Autodesk Inventor part; units mm, degrees
ref_plane "Work Plane1" through (-15.3416, 0, -12.2936) normal (1, 0, 0) x (0, 0, -1)
ref_plane "Work Plane2" through (-24.8666, 0, -12.2936) normal (1, 0, 0) x (0, 0, -1)
ref_plane "YZ Plane" through (0, 0, 0) normal (1, 0, 0) x (0, 1, 0)
sketch "Sketch1" plane through (0, 0, 0) normal (0, 1, 0) x (-1, 0, 0)
  line L0 (0, 0) -> (30.0482, 0)
  line L1 (30.0482, 0) -> (30.0482, -24.13)
  line L2 (30.0482, -24.13) -> (0, -24.13)
  line L3 (0, -24.13) -> (0, 0)
  line L4 (15.3416, -12.2936) -> (15.3416, -20.8026) construction
  line L5 (13.9319, -12.2936) -> (13.9319, -20.8026)
  line L6 (16.7513, -20.8026) -> (16.7513, -12.2936)
  arc A0 (16.7513, -12.2936) -> (13.9319, -12.2936) centre (15.3416, -12.2936) ccw
  arc A1 (13.9319, -20.8026) -> (16.7513, -20.8026) centre (15.3416, -20.8026) ccw
  line L7 (24.8666, -12.2936) -> (24.8666, -20.8026) construction
  line L8 (23.4569, -12.2936) -> (23.4569, -20.8026)
  line L9 (26.2763, -20.8026) -> (26.2763, -12.2936)
  arc A2 (26.2763, -12.2936) -> (23.4569, -12.2936) centre (24.8666, -12.2936) ccw
  arc A3 (23.4569, -20.8026) -> (26.2763, -20.8026) centre (24.8666, -20.8026) ccw
  line L10 (26.4414, -4.4958) -> (3.6068, -4.4958) construction
  line L11 (26.4414, -2.7958) -> (3.6068, -2.7958)
  line L12 (3.6068, -6.1958) -> (26.4414, -6.1958)
  arc A4 (26.4414, -6.1958) -> (26.4414, -2.7958) centre (26.4414, -4.4958) ccw
  arc A5 (3.6068, -2.7958) -> (3.6068, -6.1958) centre (3.6068, -4.4958) ccw
  point P0 (15.3416, -16.5481)
  point P1 (24.8666, -16.5481)
  point P2 (15.0241, -4.4958)
  dimension "d0" = 30.0482
  dimension "d1" = 24.13
  dimension "d5" = 12.2936
  dimension "d6" = 2.8194
  dimension "d8" = 3.3274
  dimension "d11" = 9.525
  dimension "d16" = 3.4
  dimension "d17" = 4.4958
  dimension "d18" = 3.6068
  dimension "d19" = 3.6068
  dimension "d43" = 5.1816
extrude "Shape" add sketch "Sketch1" along normal blind 2.54
sketch "Sketch2" plane through (0, 2.54, 0) normal (0, 1, 0) x (1, 0, 0)
  line L0 (0, 24.13) -> (-30.0482, 24.13)
  line L1 (0, 0) -> (0, 24.13)
  line L2 (-30.0482, 24.13) -> (0, 24.13)
  line L3 (0, 24.13) -> (0, 9.5)
  line L4 (0, 9.5) -> (-30.0482, 9.5)
  line L5 (-30.0482, 9.5) -> (-30.0482, 24.13)
  line L6 (-30.0482, 0) -> (0, 0)
  line L7 (-11.9634, 9.5) -> (-11.9634, 24.13)
  line L8 (-11.9634, 24.13) -> (-18.6944, 24.13)
  line L9 (-18.6944, 24.13) -> (-18.6944, 9.5)
  arc A0 (-16.7513, 12.2936) -> (-13.9319, 12.2936) centre (-15.3416, 12.2936) ccw
  line L10 (-18.1778, 2.3562) -> (-11.9634, 24.13) construction
  line L11 (-12.9982, 4.0205) -> (-18.6944, 24.13) construction
  line L12 (-18.6944, 9.5) -> (-1.5875, 9.5)
  line L13 (-28.2194, 24.13) -> (-28.2194, 9.5)
  line L14 (-21.4884, 9.5) -> (-21.4884, 24.13)
  line L15 (-28.2194, 9.5) -> (-11.1125, 9.5)
  line L16 (-21.4884, 24.13) -> (-28.2194, 24.13)
  point P0 (-11.9634, 24.13)
  point P1 (-21.4884, 9.5)
  point P2 (-18.6944, 9.5)
  point P3 (-28.2194, 24.13)
  dimension "d22" = 9.5
  dimension "d23" = 6.731
  dimension "d27" = 9.525
  dimension "d44" = 1.8288
extrude "Extrusion2" add sketch "Sketch2" along normal blind 3.937 contours L1 L4 L7 L0 | L9 L4 L14 L0 | L13 L4 L5 L0
ref_plane "Work Plane1" through (-15.3416, 0, -12.2936) normal (1, 0, 0) x (0, 0, -1)
ref_plane "Work Plane2" through (-24.8666, 0, -12.2936) normal (1, 0, 0) x (0, 0, -1)
sketch "Sketch3" plane through (0, 0, 0) normal (1, 0, 0) x (0, 0, -1)
  line L0 (24.13, 6.477) -> (9.5, 6.477)
  line L1 (24.13, 6.477) -> (21.59, 6.477)
  line L2 (21.59, 6.477) -> (21.59, 5.207)
  line L3 (21.59, 5.207) -> (24.13, 5.207)
  line L4 (24.13, 5.207) -> (24.13, 6.477)
  point P0 (0, 0)
  dimension "d35" = 2.54
  dimension "d36" = 1.27
extrude "Extrusion3" cut sketch "Sketch3" against normal through all
fillet "Fillet2" radius 3.175 4 edges at (0, 1.27, 0) (0, 2.6035, -24.13) (-30.0482, 2.6035, -24.13) (-30.0482, 1.27, 0)
equation "\"d19\" = d18"
equation "\"d27\" = d11"
properties part number "Limit switch mount top nut well"
CAD build for the part. Positions are in the model's coordinates, mm. A direction names the side the tool comes from. Give positions to 0.01 mm unless a question says otherwise; leave off trailing zeros. Loops run counter-clockwise (first coordinate to the right, second up) from the corner with the lowest first, then second, coordinate; pieces in that order, holes last. Notation, with made-up numbers: M -40,19 L -31,19 A22 cw -31,25 Z; hole C 33,-15 d8. An arc over 180 degrees is marked long. Write each question's results on one line, items separated by ' | '.
Q1. Band-saw the part on D-D on y = 1.25. Write the cut outline in (x, z) (3 decimals), and give its area (3 significant figures).
Geometry check:
outline: M -30.048,-20.955 A3.175 ccw -26.873,-24.13 L -3.175,-24.13 A3.175 ccw 0,-20.955 L 0,-3.175 A3.175 ccw -3.175,0 L -26.873,0 A3.175 ccw -30.048,-3.175 Z; hole M -26.441,-6.196 L -3.607,-6.196 A1.7 ccw -3.607,-2.796 L -26.441,-2.796 A1.7 ccw Z; hole M -26.276,-20.803 A1.41 ccw -23.457,-20.803 L -23.457,-12.294 A1.41 ccw -26.276,-12.294 Z; hole M -16.751,-20.803 A1.41 ccw -13.932,-20.803 L -13.932,-12.294 A1.41 ccw -16.751,-12.294 Z | area: 569 mm²
Q2. Band-saw the part on B-B on z = -16.75. Write the cut outline in (x, y).
Geometry check:
outline: M -30.05,0 L -26.28,0 L -26.28,2.54 L -28.22,2.54 L -28.22,6.48 L -30.05,6.48 Z; M -23.46,0 L -16.75,0 L -16.75,2.54 L -18.69,2.54 L -18.69,6.48 L -21.49,6.48 L -21.49,2.54 L -23.46,2.54 Z; M -13.93,0 L 0,0 L 0,6.48 L -11.96,6.48 L -11.96,2.54 L -13.93,2.54 Z
Q3. Flat gauge pins, fed straight in: P1, Ø2, axis at x = -9, z = -23, coming from the +Y side; P2, Ø0.6, axis at x = -29, y = 6, coming from the -Z side; P3, Ø1.4, axis at x = -20, y = 5, coming from the +Z side. Where does each tip first touch, or does it go through?
Geometry check:
P1: stops at y = 5.21 | P2: stops at z = -21.59 | P3: stops at z = -9.5
Q4. Band-saw the part on A-A on x = -22. Write the cut outline in (y, z), and give its area (3 significant figures).
Geometry check:
outline: M 0,-24.13 L 2.54,-24.13 L 2.54,-6.2 L 0,-6.2 Z; M 0,-2.8 L 2.54,-2.8 L 2.54,0 L 0,0 Z | area: 52.7 mm²
Q5. Mould opens along X. For faces 6 (the face through (-18.694, 4, -17)), 7 (the face through (0, 3, -14)), 8 (the face through (-29, 6.477, -16)) say: pulls with the +X half, pulls with the -X half, needs draft (parallel to the pull), parting line crosses it, or undercut.
Geometry check:
face 6: undercut | face 7: pulls with the +X half | face 8: needs draft
Q6. Band-saw the part on C-C on y = 6. Write the cut outline in (x, z) (3 decimals), and give its area (4 significant figures).
Geometry check:
outline: M -30.048,-20.955 A3.175 ccw -29.984,-21.59 L -28.219,-21.59 L -28.219,-9.5 L -30.048,-9.5 Z; M -21.488,-21.59 L -18.694,-21.59 L -18.694,-9.5 L -21.488,-9.5 Z; M -11.963,-21.59 L -0.064,-21.59 A3.175 ccw 0,-20.955 L 0,-9.5 L -11.963,-9.5 Z | area: 200.5 mm²
Q7. Which spindle directions (+Z, -Z, +X, -X, +Y, -Y) get a long thin tool onto all of the face, cutting with end or side? Do faces 1 (the face through (-6, 5.207, -23)), 2 (the face through (-13, 2, -24.13)), 3 (the face through (-20, 4, -9.5)), 4 (the face through (-28.14, 1.25, -4.46)), 5 (the face through (-11.963, 4, -17)). Say none if no direction does.
Geometry check:
face 1: -Z, +X, -X, +Y | face 2: -Z, +X, -X, +Y, -Y | face 3: +Z, +X, -X, +Y | face 4: +Y, -Y | face 5: +Z, -Z, +Y
Q8. Probe probe 1 along X at (y, z) = (5, -20.75); probe 2 along Z at (x, y) = (-9.5, 1.25); probe 3 along Y at (x, z) = (-17.5, -12.5). List the from-to ranges inside material, lowest first.
Geometry check:
probe 1: x = -30.05 to -28.22, -21.49 to -18.69, -11.96 to 0 | probe 2: z = -24.13 to -6.2, -2.8 to 0 | probe 3: y = 0 to 2.54
